Input: part model. Units: mm. Frame: model coordinates. A direction names the side the tool comes from. Round coordinates to 2 decimals unless told otherwise and drop trailing zeros. Order: outer loops, then holes, each group sorted by start corner. A loop starts at its lowest first (then second) coordinate and runs counter-clockwise, first axis right, second up. Notation, with made-up numbers: (83.25, 35.5) -> (110.25, 35.5) arc R11 ccw to (110.25, 54.5) -> close; hole circle Ø6 at (3, 63). An arc over 180 degrees is marked (long way). Answer as CSV lines item,"result". Start each with the question number.
1) First-contact query: P1, Ø8, axis at y = 22, z = 24, coming from the -X side; P2, Ø1, axis at x = 26, y = 72.5, coming from the +Z side; P3, Ø1, axis at x = 104.5, y = 25, coming from the -Z side; P4, Ø2.5, axis at y = 19.25, z = 18.5, coming from the +X side. Flat tips, straight axial feed; report the tip coordinate or a pass-through.
2) Line query: L1, parallel to Y at x = 167.5, z = 0.95; L2, parallel to Y at x = 1.4, z = 18.5; L3, parallel to X at y = 34.5, z = 19.5. Output: solid intervals per line, ascending.
3) Mould query, pull axis Z, two halves, no side actions, for faces 4 (the face through (6.684, 72.514, 23.873)), 5 (the face through (0.986, 21.233, 18.24)), 6 (the face through (2, 36, 18)). Classes: +Z half, -Z half, draft (parallel to the pull), parting line (faces both ways), or undercut.
4) Section query C-C, the plane x = 86. Output: boundary loops of the cut face in (y, z), and give its area (3 significant figures).
5) Section query D-D, the plane y = 30. Output: boundary loops of the cut face in (x, z), and give its area (3 significant figures).
6) Section query B-B, the plane z = 11.5. Output: boundary loops of the cut face in (x, y).
7) Section query A-A, the plane y = 19.25. Output: boundary loops of the cut face in (x, z), and give its area (3 significant figures).
8) Access query for faces 1 (the face through (138.35, 4.39, 25.42)), 2 (the face through (138.35, 2.33, 25.53)), 3 (the face through (193, 36, 18)). Directions: +Z, -Z, +X, -X, +Y, -Y. A direction counts if a zero-diameter tool reaches every point of the face in a straight line with its end or side. Return the directions, or none.
```python
from build123d import *

# Parameters (mm, degrees)
SKETCH1_W            = 195
SKETCH1_H            = 73.5
SKETCH1_R            = 1.6
BOSS_EXTRUDE1_DEPTH  = 2
SKETCH2_W            = 2
SKETCH2_H            = 73.5
BOSS_EXTRUDE2_DEPTH  = 32
BOSS_EXTRUDE3_DEPTH  = 2
BOSS_EXTRUDE4_DEPTH  = 50
MIRROR3_COPY_1_DEPTH = 50
FILLET1_R            = 5
SKETCH6_R            = 1
BOSS_EXTRUDE5_DEPTH  = 15
SKETCH7_R            = 2
CUT_EXTRUDE1_DEPTH   = 212.147460321


with BuildPart() as part:
    # Sketch1 → Boss-Extrude1 (new body)
    with BuildSketch(Plane.XY):
        with Locations((97.5, 36.75)):
            Rectangle(SKETCH1_W, SKETCH1_H)
        with Locations((27.5, 67.364107359)):
            Circle(SKETCH1_R, mode=Mode.SUBTRACT)
        with Locations((97.5, 67.364107359)):
            Circle(SKETCH1_R, mode=Mode.SUBTRACT)
        with Locations((167.5, 67.364107359)):
            Circle(SKETCH1_R, mode=Mode.SUBTRACT)
        with Locations(Location((167.5, 6.135892641, 0), (0, 0, 180))):
            Circle(SKETCH1_R, mode=Mode.SUBTRACT)
        with Locations(Location((97.5, 6.135892641, 0), (0, 0, 180))):
            Circle(SKETCH1_R, mode=Mode.SUBTRACT)
        with Locations(Location((27.5, 6.135892641, 0), (0, 0, 180))):
            Circle(SKETCH1_R, mode=Mode.SUBTRACT)
    extrude(amount=BOSS_EXTRUDE1_DEPTH)

    # Sketch2 → Boss-Extrude2 (add)
    with BuildSketch(Plane.XY.offset(2)):
        with Locations((1, 36.75)):
            Rectangle(SKETCH2_W, SKETCH2_H)
        with Locations((194, 36.75)):
            Rectangle(SKETCH2_W, SKETCH2_H)
    extrude(amount=BOSS_EXTRUDE2_DEPTH)

    # Sketch3 → Boss-Extrude3 (add)
    with BuildSketch(Plane.XZ):
        Polygon((0, 0), (0, 29), (2, 29), (11.5, 18.6), (183.5, 18.6), (193, 26.325039357), (195, 26.325039357), (195, 0), align=None)
    boss_extrude3 = extrude(amount=-BOSS_EXTRUDE3_DEPTH)

    # Mirror1: Boss-Extrude3 across plane
    add(boss_extrude3.mirror(Plane(origin=(0, 36.75, 0), x_dir=(0, 0, 1), z_dir=(0, -1, 0))))

    # 3DSketch1 → Boss-Extrude4 (add)
    with BuildSketch(Plane(origin=(32, 0, 18.6), x_dir=(0, 0.995265198446773, -0.09719662936905633), z_dir=(1, 0, 0))):
        with BuildLine():
            Line((0, 0), (1.990530397, 0.194393259))
            ThreePointArc((1.990530397, 0.194393259), (3.755453085, 7.307606505), (8.506639352, 12.887838028))
            Line((8.506639352, 12.887838028), (6.133305317, 12.656060539))
            ThreePointArc((6.133305317, 12.656060539), (1.603781504, 7.03695825), (0, 0))
        make_face()
    boss_extrude4 = extrude(amount=BOSS_EXTRUDE4_DEPTH)

    # Mirror2: Boss-Extrude4 across plane
    add(boss_extrude4.mirror(Plane(origin=(97.5, 0, 0), x_dir=(0, 0, 1), z_dir=(1, 0, 0))))

    # Mirror3: Boss-Extrude4 across plane
    add(boss_extrude4.mirror(Plane(origin=(0, 36.75, 0), x_dir=(0, 0, 1), z_dir=(0, -1, 0))))

    # Mirror3 copy 1 sketch → Mirror3 copy 1 (add)
    with BuildSketch(Plane(origin=(163, 73.5, 18.6), x_dir=(0, -0.995265198446773, -0.09719662936905633), z_dir=(-1, 0, 0))):
        with BuildLine():
            Line((0, 0), (1.990530397, 0.194393259))
            ThreePointArc((1.990530397, 0.194393259), (3.755453085, 7.307606505), (8.506639352, 12.887838028))
            Line((8.506639352, 12.887838028), (6.133305317, 12.656060539))
            ThreePointArc((6.133305317, 12.656060539), (1.603781504, 7.03695825), (0, 0))
        make_face()
    extrude(amount=MIRROR3_COPY_1_DEPTH)

    # Fillet1
    fillet1_edges = [part.edges().sort_by_distance(p)[0] for p in [
        (1, 0, 34),
        (1, 73.5, 34),
        (194, 73.5, 34),
        (194, 0, 34),
    ]]
    fillet(fillet1_edges, radius=FILLET1_R)

    # Sketch6 → Boss-Extrude5 (add)
    with BuildSketch(Plane.ZY):
        with Locations(Location((5, 46.75, 0), (0, 0, 180))):
            Circle(SKETCH6_R)
        with Locations(Location((5, 26.75, 0), (0, 0, 180))):
            Circle(SKETCH6_R)
    extrude(amount=BOSS_EXTRUDE5_DEPTH)

    # Sketch7 → Cut-Extrude1 (cut, through all)
    with BuildSketch(Plane.ZY):
        with Locations((18.5, 54.25)):
            Circle(SKETCH7_R)
        with Locations((18.5, 19.25)):
            Circle(SKETCH7_R)
    extrude(amount=-CUT_EXTRUDE1_DEPTH, mode=Mode.SUBTRACT)


solid = part.part
```
Findings:
1,P1,"stops at x = 0"
1,P2,"stops at z = 18.6"
1,P3,"stops at z = 0"
1,P4,"passes through"
2,L1,"y = 0 to 4.54, 7.74 to 65.76, 68.96 to 73.5"
2,L2,"y = 0 to 17.25, 21.25 to 52.25, 56.25 to 73.5"
2,L3,"x = 0 to 2, 193 to 195"
3,face 4,"+Z half"
3,face 5,"undercut"
3,face 6,"draft"
4,outline,"(0, 0) -> (73.5, 0) -> (73.5, 18.6) -> (71.5, 18.6) -> (71.5, 2) -> (2, 2) -> (2, 18.6) -> (0, 18.6) -> close"
4,area,"213 mm^2"
5,outline,"(0, 0) -> (195, 0) -> (195, 34) -> (193, 34) -> (193, 2) -> (2, 2) -> (2, 34) -> (0, 34) -> close"
5,area,"518 mm^2"
6,outline,"(0, 0) -> (195, 0) -> (195, 73.5) -> (0, 73.5) -> close; hole (2, 2) -> (193, 2) -> (193, 71.5) -> (2, 71.5) -> close"
7,outline,"(0, 0) -> (195, 0) -> (195, 16.5) -> (193, 16.5) -> (193, 2) -> (2, 2) -> (2, 16.5) -> (0, 16.5) -> close; (0, 20.5) -> (2, 20.5) -> (2, 34) -> (0, 34) -> close; (193, 20.5) -> (195, 20.5) -> (195, 34) -> (193, 34) -> close"
7,area,"502 mm^2"
8,face 1,"none"
8,face 2,"+Z, -Y"
8,face 3,"+Z"
